Design review of the part built by this model. Coordinates are the model's own, in mm. Face numbers are marked on the shaded views. A direction names the side the tool comes from. Round coordinates to 2 decimals unless told otherwise and drop trailing zeros. Write each loop counter-clockwise with the first axis right and the second up, starting at its lowest first coordinate (ties: lowest second). Pieces come first, ordered by that corner, then holes. Notation, with made-up numbers: M -11,-32 L -6,-32 A20 ccw -6,3 Z; hole C 17,78 d6. An arc over 180 degrees is marked long. One line per question, with ' | ' between items. Start each with the question number.
Item 1: Add section B-B, the plane x = -21. State the section outline as (y, z) points, and give its area (3 significant figures).
Item 2: Add section C-C, the plane z = 17. State the section outline as (x, y) points, and give its area (4 significant figures).
Item 3: Machinability: for the marked faces 1, 2 and 3, which of the approach directions +Z, -Z, +X, -X, +Y, -Y give a long, thin tool a straight path to every point of the face, cutting with its end or side? Answer none if there is none.
Item 4: Add section D-D, the plane z = 3.5. State the section outline as (x, y) points, and give its area (3 significant figures).
Item 5: Insertion check: pin 1 Ø1 at (y, z) = (-20.5, 17) entering from -X; pin 2 Ø3 at (x, z) = (-3.5, -7) entering from +Y; pin 3 Ø4 at (y, z) = (-7, 5.5) entering from +X; pin 4 Ø12 at (x, y) = (21, -20.5) entering from +Z. Each pin has a flat end and moves straight along its axis. Give the tip position at first contact, or say it passes through.
Item 6: For L1, parallel to Y at x = 9.5, z = -9.5; L2, parallel to Z at x = -18, y = -15; L3, parallel to X at y = -15.5, z = 11, list the stretches that pass through material, from the lowest coordinate up.
Item 7: Add section A-A, the plane y = -13.5. State the section outline as (x, z) points (3 decimals).
Item 8: Draft analysis for pull direction X (two halves, no side actions). For the marked faces 4, 5 and 6, state which applies: released by +X, released by -X, zero draft, split by the parting line, or undercut.
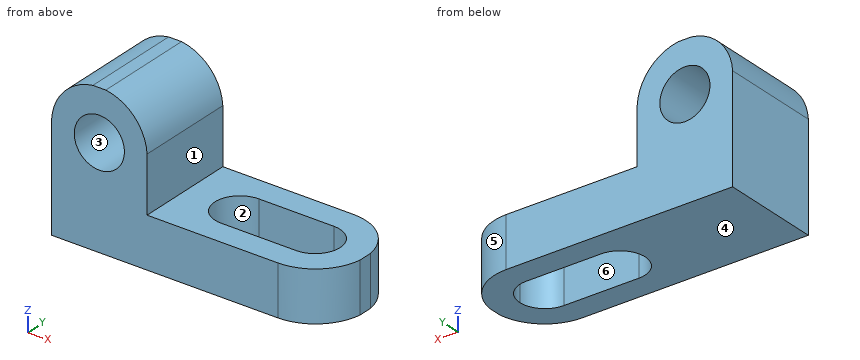
```python
from build123d import *

# Parameters (mm, degrees)
F1_DEPTH = 25.4
F3_DEPTH = 25.401
F5_DEPTH = 12.701


with BuildPart() as f1:
    # F0 (on Front) → F1 (new body)
    with BuildSketch(Plane.XZ):
        Polygon((-6.2236683385, 24.0342710525), (-30.4063118957, 24.0342710525), (-30.4063118957, -14.0657289475), (39.4436881043, -14.0657289475), (39.4436881043, -1.3657289475), (-6.2236683385, -1.3657289475), align=None)
    extrude(amount=F1_DEPTH)

    # F2 (on face) → F3 (cut, through all)
    with BuildSketch(Plane.XZ.offset(25.4)):
        with BuildLine():
            ThreePointArc((-24.6649901171, 11.3342710525), (-18.3149901171, 4.9842710525), (-11.9649901171, 11.3342710525))
            Line((-11.9649901171, 11.3342710525), (-24.6649901171, 11.3342710525))
        make_face()
        with BuildLine():
            Line((-24.6649901171, 11.3342710525), (-11.9649901171, 11.3342710525))
            ThreePointArc((-11.9649901171, 11.3342710525), (-18.3149901171, 17.6842710525), (-24.6649901171, 11.3342710525))
        make_face()
        with BuildLine():
            Line((-6.2236683385, 12.7333663785), (-6.2236683385, 11.3342710525))
            ThreePointArc((-6.2236683385, 11.3342710525), (-6.2034489564, 12.0338187155), (-6.2236683385, 12.7333663785))
        make_face()
        with BuildLine():
            ThreePointArc((-16.678355462, 24.0342710525), (-9.4244440948, 20.258636082), (-6.2236683385, 12.7333663785))
            Line((-6.2236683385, 12.7333663785), (-6.2236683385, 24.0342710525))
            Line((-6.2236683385, 24.0342710525), (-16.678355462, 24.0342710525))
        make_face()
        with BuildLine():
            ThreePointArc((-30.4063118957, 12.7333663785), (-30.4265312777, 12.0338187155), (-30.4063118957, 11.3342710525))
            Line((-30.4063118957, 11.3342710525), (-30.4063118957, 12.7333663785))
        make_face()
        with BuildLine():
            Line((-19.9516247721, 24.0342710525), (-16.678355462, 24.0342710525))
            ThreePointArc((-16.678355462, 24.0342710525), (-18.3149901171, 24.1453598762), (-19.9516247721, 24.0342710525))
        make_face()
        with BuildLine():
            Line((-30.4063118957, 24.0342710525), (-30.4063118957, 12.7333663785))
            ThreePointArc((-30.4063118957, 12.7333663785), (-27.2055361393, 20.258636082), (-19.9516247721, 24.0342710525))
            Line((-19.9516247721, 24.0342710525), (-30.4063118957, 24.0342710525))
        make_face()
    extrude(amount=-F3_DEPTH, mode=Mode.SUBTRACT)

    # F4 (on face) → F5 (cut, through all)
    with BuildSketch(Plane.XY.offset(-1.3657289475)):
        with BuildLine():
            ThreePointArc((33.0936881043, -12.7), (31.2338161649, -8.2098719395), (26.7436881043, -6.35))
            Line((26.7436881043, -6.35), (26.7436881043, -19.05))
            ThreePointArc((26.7436881043, -19.05), (31.2338161649, -17.1901280605), (33.0936881043, -12.7))
        make_face()
        with BuildLine():
            Line((26.7436881043, -19.05), (26.7436881043, -6.35))
            ThreePointArc((26.7436881043, -6.35), (20.3936881043, -12.7), (26.7436881043, -19.05))
        make_face()
        with BuildLine():
            ThreePointArc((26.7436881043, -19.05), (20.3936881043, -12.7), (26.7436881043, -6.35))
            Line((26.7436881043, -6.35), (7.6936881043, -6.35))
            ThreePointArc((7.6936881043, -6.35), (12.1838161649, -8.2098719395), (14.0436881043, -12.7))
            ThreePointArc((14.0436881043, -12.7), (12.1838161649, -17.1901280605), (7.6936881043, -19.05))
            Line((7.6936881043, -19.05), (26.7436881043, -19.05))
        make_face()
        with BuildLine():
            Line((39.4436881043, 0), (26.981144502, 0))
            ThreePointArc((26.981144502, 0), (35.251198478, -3.1641502734), (39.4436881043, -10.9634239866))
            Line((39.4436881043, -10.9634239866), (39.4436881043, 0))
        make_face()
        with BuildLine():
            ThreePointArc((14.0436881043, -12.7), (12.1838161649, -8.2098719395), (7.6936881043, -6.35))
            Line((7.6936881043, -6.35), (7.6936881043, -19.05))
            ThreePointArc((7.6936881043, -19.05), (12.1838161649, -17.1901280605), (14.0436881043, -12.7))
        make_face()
        with BuildLine():
            Line((7.6936881043, -19.05), (7.6936881043, -6.35))
            ThreePointArc((7.6936881043, -6.35), (1.3436881043, -12.7), (7.6936881043, -19.05))
        make_face()
        with BuildLine():
            ThreePointArc((39.4436881043, -14.4365760134), (39.5629712668, -12.7), (39.4436881043, -10.9634239866))
            Line((39.4436881043, -10.9634239866), (39.4436881043, -14.4365760134))
        make_face()
        with BuildLine():
            Line((39.4436881043, -25.4), (39.4436881043, -14.4365760134))
            ThreePointArc((39.4436881043, -14.4365760134), (35.251198478, -22.2358497266), (26.981144502, -25.4))
            Line((26.981144502, -25.4), (39.4436881043, -25.4))
        make_face()
    extrude(amount=-F5_DEPTH, mode=Mode.SUBTRACT)


solid = f1.part
```
Computed values:
1) outline: M -25.4,-14.07 L 0,-14.07 L 0,5.58 L -25.4,5.58 Z; M -25.4,17.09 L 0,17.09 L 0,23.84 L -25.4,23.84 Z | area: 671 mm^2
2) outline: M -29.36,-25.4 L -21.18,-25.4 L -21.18,0 L -29.36,0 Z; M -15.45,-25.4 L -7.27,-25.4 L -7.27,0 L -15.45,0 Z | area: 415.5 mm^2
3) face 1: +Z, +X, +Y, -Y | face 2: +Z, -Z | face 3: +Y, -Y
4) outline: M -30.41,-25.4 L -6.22,-25.4 L -6.22,0 L -30.41,0 Z | area: 614 mm^2
5) pin 1: stops at x = -29.57 | pin 2: stops at y = 0 | pin 3: stops at x = -6.22 | pin 4: stops at z = -1.37
6) L1: y = -25.4 to -19.05, -6.35 to 0 | L2: z = -14.07 to 4.99, 17.68 to 24.03 | L3: x = -30.41 to -24.66, -11.97 to -6.22
7) outline: M -30.406,-14.066 L 1.394,-14.066 L 1.394,-1.366 L -6.224,-1.366 L -6.224,12.733 A12.112 ccw -16.678,24.034 L -19.952,24.034 A12.112 ccw -30.406,12.733 Z; M 33.043,-14.066 L 39.444,-14.066 L 39.444,-1.366 L 33.043,-1.366 Z; hole C -18.315,11.334 d12.7
8) face 4: zero draft | face 5: released by +X | face 6: undercut
